from build123d import *

# Parameters (mm, degrees)
SKETCH1_R           = 2
SKETCH1_R_2         = 9.5
BOSS_EXTRUDE1_DEPTH = 3
FILLET1_R           = 10


with BuildPart() as part:
    # Sketch1 → Boss-Extrude1 (new, symmetric)
    with BuildSketch(Plane.XY):
        with BuildLine():
            Line((15, 60), (-15, 60))
            Line((-15, 60), (-15, 16.770509831))
            ThreePointArc((-15, 16.770509831), (0, -22.5), (15, 16.770509831))
            Line((15, 16.770509831), (15, 60))
        make_face()
        with Locations((0, 33)):
            Circle(SKETCH1_R, mode=Mode.SUBTRACT)
        with Locations((0, 55)):
            Circle(SKETCH1_R, mode=Mode.SUBTRACT)
        with Locations((17.5, 0)):
            Circle(SKETCH1_R, mode=Mode.SUBTRACT)
        with Locations((-17.5, 0)):
            Circle(SKETCH1_R, mode=Mode.SUBTRACT)
        with Locations((0, -17.5)):
            Circle(SKETCH1_R, mode=Mode.SUBTRACT)
        Circle(SKETCH1_R_2, mode=Mode.SUBTRACT)
        with Locations((0, 17.5)):
            Circle(SKETCH1_R, mode=Mode.SUBTRACT)
    extrude(amount=BOSS_EXTRUDE1_DEPTH, both=True)

    # Fillet1
    fillet1_edges = [part.edges().sort_by_distance(p)[0] for p in [
        (-15, 60, 0),
        (15, 60, 0),
        (15, 16.770509831, 0),
        (-15, 16.770509831, 0),
    ]]
    fillet(fillet1_edges, radius=FILLET1_R)


solid = part.part
Check sheet for the modelled part. Datum: model origin and axes. Units: mm. A direction names the side the tool comes from. Round coordinates to 2 decimals unless told otherwise and drop trailing zeros. Order: outer loops, then holes, each group sorted by start corner. A loop starts at its lowest first (then second) coordinate and runs counter-clockwise, first axis right, second up. Notation, with made-up numbers: M 42.5,13 L 88.5,13 A12 cw 88.5,32 Z; hole C 53,-34 d7. An arc over 180 degrees is marked long. One line per item, written item: value. Start each with the question number.
1. Section check C-C on z = 0.85. Enter the section's corners in (x, y), and give its area (3 significant figures).
2. Section check A-A on x = 0. Enter the section's corners in (y, z).
3. Section check B-B on y = 33. Enter the section's corners in (x, z), and give its area (3 significant figures).
4. Scan lines: line 1 along Y through (x, z) = (0, 1.5); line 2 along X through (y, z) = (-7.5, 0.65); line 3 along X through (y, z) = (45.5, -0.2). Record each from-to range of solid material in increasing order.
5. Release check for a two-part mould opening along X. For faces 1 (the cylindrical face through (-19.1, -1.2, 0)), 2 (the cylindrical face through (-0.71, -22.49, 0.04)), 3 (the cylindrical face through (-11.99, 57.15, 0.04)), 4 (the cylindrical face through (11.99, 57.15, -0.04)) record: released by +X, released by -X, zero draft, split by the parting line, or undercut.
6. Section check D-D on y = 0. Enter the section's corners in (x, z), and give its area (3 significant figures).
7. Access from +Z, -Z, +X, -X, +Y, -Y to the whole of each face (thin tool, end or side, straight path). Record for faces 5 (the flat face through (15, 35, 0)), 6 (the flat face through (-15, 36, 0)), 7 (the cylindrical face through (-0.26, -15.517, -0.042)).
8. Gauge pin test, flat ends, axial feed: P1, Ø1.8, axis at y = 28.5, z = 1.5, coming from the +X side; P2, Ø2, axis at x = -7.5, z = -1.5, coming from the +Y side. Record the tip position at first contact, or that the pin passes through.
Results found:
1. outline: M -17.31,14.38 A22.5 ccw long 17.31,14.38 A10 cw 15,20.77 L 15,50 A10 ccw 5,60 L -5,60 A10 ccw -15,50 L -15,20.77 A10 cw Z; hole C -17.5,0 d4; hole C 0,0 d19; hole C 0,-17.5 d4; hole C 0,17.5 d4; hole C 0,33 d4; hole C 0,55 d4; hole C 17.5,0 d4
1. area: 2,370 mm^2
2. outline: M -22.5,-3 L -19.5,-3 L -19.5,3 L -22.5,3 Z; M -15.5,-3 L -9.5,-3 L -9.5,3 L -15.5,3 Z; M 9.5,-3 L 15.5,-3 L 15.5,3 L 9.5,3 Z; M 19.5,-3 L 31,-3 L 31,3 L 19.5,3 Z; M 35,-3 L 53,-3 L 53,3 L 35,3 Z; M 57,-3 L 60,-3 L 60,3 L 57,3 Z
3. outline: M -15,-3 L -2,-3 L -2,3 L -15,3 Z; M 2,-3 L 15,-3 L 15,3 L 2,3 Z
3. area: 156 mm^2
4. line 1: -22.5 to -19.5, -15.5 to -9.5, 9.5 to 15.5, 19.5 to 31, 35 to 53, 57 to 60
4. line 2: -21.21 to -5.83, 5.83 to 21.21
4. line 3: -15 to 15
5. face 1: undercut
5. face 2: split by the parting line
5. face 3: released by -X
5. face 4: released by +X
6. outline: M -22.5,-3 L -19.5,-3 L -19.5,3 L -22.5,3 Z; M -15.5,-3 L -9.5,-3 L -9.5,3 L -15.5,3 Z; M 9.5,-3 L 15.5,-3 L 15.5,3 L 9.5,3 Z; M 19.5,-3 L 22.5,-3 L 22.5,3 L 19.5,3 Z
6. area: 108 mm^2
7. face 5: +Z, -Z, +X, +Y
7. face 6: +Z, -Z, -X, +Y
7. face 7: +Z, -Z
8. P1: x = 15
8. P2: y = 59.89
